from build123d import *

# Parameters (mm, degrees)
SKETCH1_W           = 17.78
SKETCH1_H           = 17.78
BOSS_EXTRUDE1_DEPTH = 2.54
SKETCH2_R           = 1.4732
CUT_EXTRUDE1_DEPTH  = 3.54
FILLET1_R           = 2.54


with BuildPart() as part:
    # Sketch1 → Boss-Extrude1 (new body)
    with BuildSketch(Plane(origin=(0, 0, 0), x_dir=(1, 0, 0), z_dir=(0, 1, 0))):
        Rectangle(SKETCH1_W, SKETCH1_H)
    extrude(amount=BOSS_EXTRUDE1_DEPTH)

    # Sketch2 → Cut-Extrude1 (cut, through all)
    with BuildSketch(Plane(origin=(0, 2.54, 0), x_dir=(1, 0, 0), z_dir=(0, 1, 0))):
        with Locations((-4.8768, 5.3848)):
            Circle(SKETCH2_R)
        with Locations((-4.8768, -5.3848)):
            Circle(SKETCH2_R)
        with Locations((4.8768, -5.3848)):
            Circle(SKETCH2_R)
        with Locations((4.8768, 5.3848)):
            Circle(SKETCH2_R)
    extrude(amount=-CUT_EXTRUDE1_DEPTH, mode=Mode.SUBTRACT)

    # Fillet1
    fillet1_edges = [part.edges().sort_by_distance(p)[0] for p in [
        (8.89, 1.27, 8.89),
        (-8.89, 1.27, 8.89),
        (-8.89, 1.27, -8.89),
        (8.89, 1.27, -8.89),
    ]]
    fillet(fillet1_edges, radius=FILLET1_R)


solid = part.part
Can you work these out from the model? Positions are in its coordinate system, mm. Give positions to 0.01 mm unless a question says otherwise; leave off trailing zeros. Loops run counter-clockwise (first coordinate to the right, second up) from the corner with the lowest first, then second, coordinate; pieces in that order, holes last. Notation, with made-up numbers: (86, 42) -> (104, 42) arc R13 cw to (104, 51) -> close; hole circle Ø9 at (-2, 76.5). An arc over 180 degrees is marked (long way). Use one line per item in the form item = value.
1) If we section it at B-B (z = -4.75): Please give me the cut outline in (x, y), plus the area to 3 significant figures.
Answers:
outline = (-8.89, 0) -> (-6.21, 0) -> (-6.21, 2.54) -> (-8.89, 2.54) -> close; (-3.55, 0) -> (3.55, 0) -> (3.55, 2.54) -> (-3.55, 2.54) -> close; (6.21, 0) -> (8.89, 0) -> (8.89, 2.54) -> (6.21, 2.54) -> close
area = 31.7 mm²
2) If we section it at C-C (y = 1.15): Please give me the cut outline in (x, z).
Answers:
outline = (-8.89, -6.35) arc R2.54 ccw to (-6.35, -8.89) -> (6.35, -8.89) arc R2.54 ccw to (8.89, -6.35) -> (8.89, 6.35) arc R2.54 ccw to (6.35, 8.89) -> (-6.35, 8.89) arc R2.54 ccw to (-8.89, 6.35) -> close; hole circle Ø2.95 at (-4.88, -5.38); hole circle Ø2.95 at (-4.88, 5.38); hole circle Ø2.95 at (4.88, -5.38); hole circle Ø2.95 at (4.88, 5.38)
3) Will this pin go through, and if not, where does the flat tip stop? pin 1 (2.5 mm diameter, centred on x = 4.88, z = -5.38, fed in from -Y) (1 decimal).
Answers:
pin_1 = through
4) I need wall thicknesses on line 1 along Z through (x, y) = (-4.75, 1.4); line 2 along Z through (x, y) = (4.5, 1.6); line 3 along X through (y, z) = (0.65, -5). Which ranges of each line are inside material? Lowest first, please.
Answers:
line_1 = -8.89 to -6.85, -3.92 to 3.92, 6.85 to 8.89
line_2 = -8.89 to -6.81, -3.96 to 3.96, 6.81 to 8.89
line_3 = -8.89 to -6.3, -3.45 to 3.45, 6.3 to 8.89
5) We'd pull the mould along X, two halves only. Please class faces 1 (the face through (-8.89, 1, 0)), 2 (the face through (0, 2.54, 0)), 3 (the face through (3.79, 1.29, -6.38)): released by +X, released by -X, zero draft, split by the parting line, or undercut.
Answers:
face_1 = released by -X
face_2 = zero draft
face_3 = undercut
6) If we section it at A-A (x = 3.75): Please give me the cut outline in (y, z), plus the area to 3 significant figures.
Answers:
outline = (0, -8.89) -> (2.54, -8.89) -> (2.54, -6.33) -> (0, -6.33) -> close; (0, -4.44) -> (2.54, -4.44) -> (2.54, 4.44) -> (0, 4.44) -> close; (0, 6.33) -> (2.54, 6.33) -> (2.54, 8.89) -> (0, 8.89) -> close
area = 35.5 mm²
